Geometry check sheet. Reference: the model listing, model coordinates, mm. Coordinates: 2 decimals unless noted, no trailing zeros. Write each loop counter-clockwise with the first axis right and the second up, starting at its lowest first coordinate (ties: lowest second). Pieces come first, ordered by that corner, then holes.
from build123d import *

# Parameters (mm, degrees)
SKETCH1_R           = 9.525
SKETCH1_R_2         = 7.874
BOSS_EXTRUDE1_DEPTH = 228.6
SKETCH2_R           = 3
CUT_EXTRUDE1_DEPTH  = 138.80592
SKETCH3_R           = 3
CUT_EXTRUDE2_DEPTH  = 138.80592


with BuildPart() as part:
    # Sketch1 → Boss-Extrude1 (new body)
    with BuildSketch(Plane.XY):
        Circle(SKETCH1_R)
        Circle(SKETCH1_R_2, mode=Mode.SUBTRACT)
    extrude(amount=BOSS_EXTRUDE1_DEPTH)

    # Sketch2 → Cut-Extrude1 (cut)
    with BuildSketch(Plane(origin=(0, 9.525, 0), x_dir=(1, 0, 0), z_dir=(0, 1, 0))):
        with Locations((0, -222.25)):
            Circle(SKETCH2_R)
    extrude(amount=-CUT_EXTRUDE1_DEPTH, mode=Mode.SUBTRACT)

    # Sketch3 → Cut-Extrude2 (cut)
    with BuildSketch(Plane(origin=(9.525, 0, 0), x_dir=(0, 0, -1), z_dir=(1, 0, 0))):
        with Locations((-6.35, 0)):
            Circle(SKETCH3_R)
    extrude(amount=-CUT_EXTRUDE2_DEPTH, mode=Mode.SUBTRACT)


solid = part.part
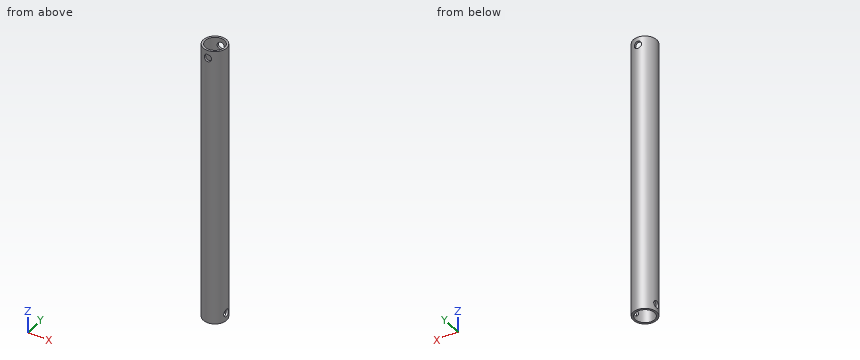
1. Sectioned sample at B-B, the plane x = 0. Record the boundary of the cut face in (y, z) (3 decimals).
Computed values:
outline: (-9.525, 0) - (-7.874, 0) - (-7.874, 219.25) - (-9.525, 219.25) - close; (-9.525, 225.25) - (-7.874, 225.25) - (-7.874, 228.6) - (-9.525, 228.6) - close; (7.874, 0) - (9.525, 0) - (9.525, 219.25) - (7.874, 219.25) - close; (7.874, 225.25) - (9.525, 225.25) - (9.525, 228.6) - (7.874, 228.6) - close
2. Thickness scan on line 1 along X through (y, z) = (0, 112.5) (3 decimals); line 2 along Z through (x, y) = (0, -8.2); line 3 along Y through (x, z) = (0.5, 14.5). Record the ranges inside material, lowest first.
Computed values:
line 1: x = -9.525 to -7.874, 7.874 to 9.525
line 2: z = 0 to 219.25, 225.25 to 228.6
line 3: y = -9.51 to -7.86, 7.86 to 9.51
3. Sectioned sample at D-D, the plane z = 148. Record the boundary of the cut face in (x, y) (3 decimals), and give its area (3 significant figures).
Computed values:
outline: circle Ø19.05 at (0, 0); hole circle Ø15.748 at (0, 0)
area: 90.2 mm2
4. Sectioned sample at C-C, the plane z = 222.25. Record the boundary of the cut face in (x, y) (3 decimals).
Computed values:
outline: (-3, -9.04) - (-3, -7.28) arc R7.874 cw to (-3, 7.28) - (-3, 9.04) arc R9.525 ccw to start; (3, -9.04) arc R9.525 ccw to (3, 9.04) - (3, 7.28) arc R7.874 cw to (3, -7.28) - close
5. Gauge pin test, flat ends, axial feed: pin 1 Ø10 at (x, z) = (-1.5, 146.5) entering from -Y (3 decimals); pin 2 Ø4 at (x, z) = (-6, 135.5) entering from +Y. Record the tip position at first contact, or that the pin passes through.
Computed values:
pin 1: stops at y = -9.525
pin 2: stops at y = 8.64
6. Sectioned sample at A-A, the plane y = 0. Record the boundary of the cut face in (x, z) (3 decimals), and give its area (3 significant figures).
Computed values:
outline: (-9.525, 0) - (-7.874, 0) - (-7.874, 3.35) - (-9.525, 3.35) - close; (-9.525, 9.35) - (-7.874, 9.35) - (-7.874, 228.6) - (-9.525, 228.6) - close; (7.874, 0) - (9.525, 0) - (9.525, 3.35) - (7.874, 3.35) - close; (7.874, 9.35) - (9.525, 9.35) - (9.525, 228.6) - (7.874, 228.6) - close
area: 735 mm2
